Here's the drawing with two shaded views (mm, measured from the low corner). I have some questions. Round coordinates to 2 decimals unless told otherwise and drop trailing zeros. Order: outer loops, then holes, each group sorted by start corner. A loop starts at its lowest first (then second) coordinate and runs counter-clockwise, first axis right, second up. Notation, with made-up numbers: (57.25, 10.25) -> (77.25, 10.25) arc R9 ccw to (77.25, 19.25) -> close; hole circle Ø3 at (52, 53.25). An arc over 180 degrees is marked (long way). Answer in a Markdown table with one row per item.
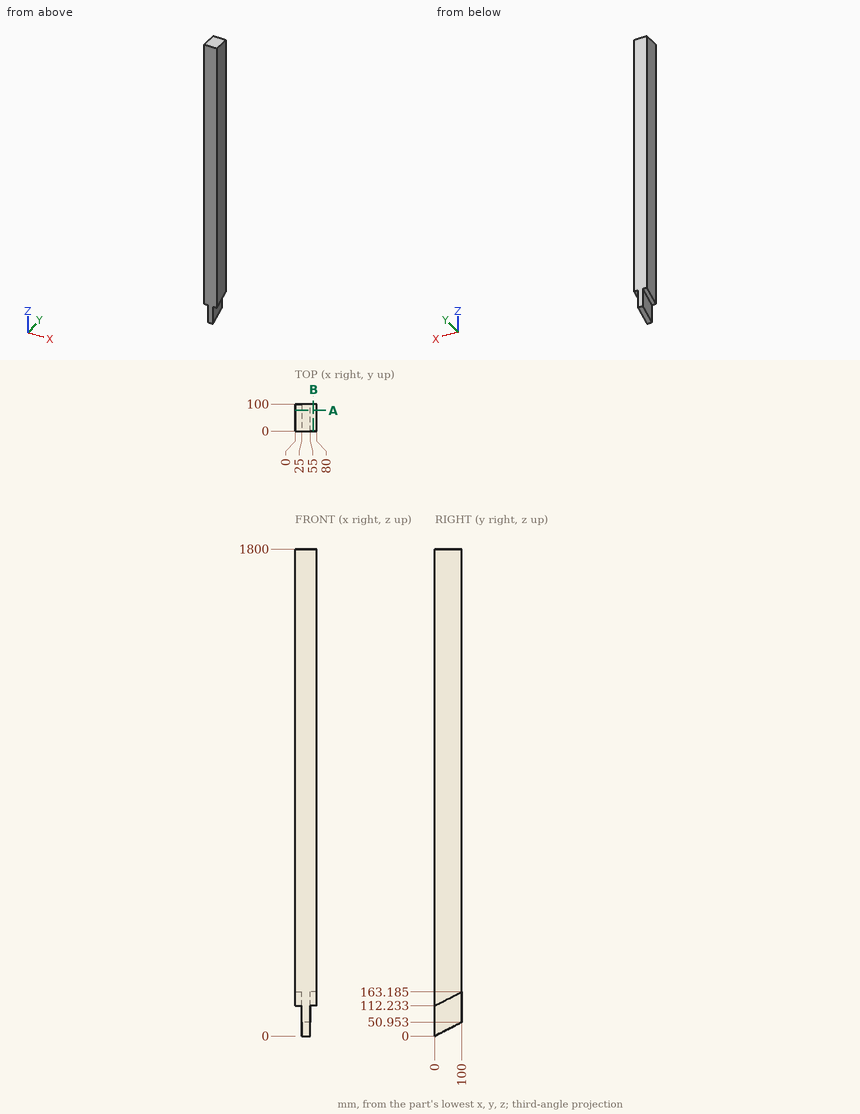
1. Please list where these lines run through material, in increasing order: line 1 along X through (y, z) = (29, 117.5); line 2 along Z through (x, y) = (54, 88.5); line 3 along Z through (x, y) = (31.5, 82).
Numbers:
| item | result |
|---|---|
| line 1 | x = 25 to 55 |
| line 2 | z = 45.09 to 1800 |
| line 3 | z = 41.78 to 1800 |
2. Suppose I cut it at A-A on y = 76. Write out the boundary of the cut face in (x, z).
Numbers:
| item | result |
|---|---|
| outline | (0, 150.96) -> (25, 150.96) -> (25, 38.72) -> (55, 38.72) -> (55, 150.96) -> (80, 150.96) -> (80, 1800) -> (0, 1800) -> close |
3. For pin 1 Ø5 at (x, y) = (29.5, 89) entering from -Z (1 decimal), with a flat end and sliding along its axis, tell me the tip position at first contact or that it passes through.
Numbers:
| item | result |
|---|---|
| pin 1 | stops at z = 44.1 |
4. Suppose I cut it at B-B on x = 67.5. Write out the boundary of the cut face in (y, z) (1 decimal), then the cut area to 3 significant figures.
Numbers:
| item | result |
|---|---|
| outline | (0, 112.2) -> (100, 163.2) -> (100, 1800) -> (0, 1800) -> close |
| area | 166,000 mm2 |
